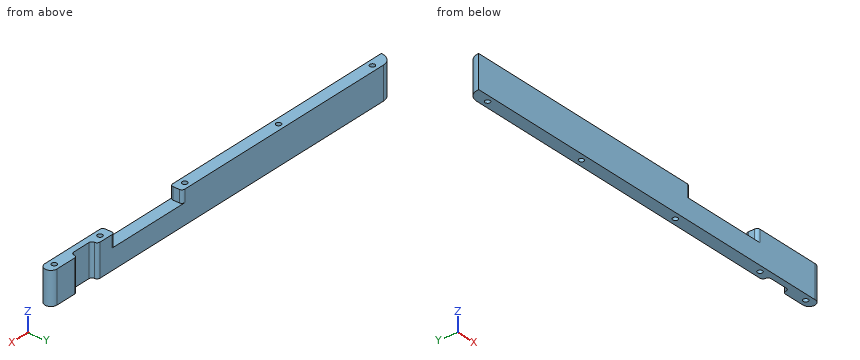
```python
from build123d import *

# Parameters (mm, degrees)
EXTRUDE_854_DEPTH      = 8
SKETCH_2_W             = 20
SKETCH_2_H             = 3
CUT_EXTRUDE_1137_DEPTH = 3
HOLE_WIZARD_1_6_D      = 1.25
SKETCH_7_W             = 6
SKETCH_7_H             = 1.5
CUT_EXTRUDE_2764_DEPTH = 102.181383663
FILLET_2_RADIUS        = 1.5
FILLET_2_LENGTH        = 8
FILLET_3_R             = 0.75


with BuildPart() as part:
    # Model → Extrude 854 (new body)
    with BuildSketch(Plane.XY):
        with BuildLine():
            Line((100.82, 3), (3, 3))
            ThreePointArc((3, 3), (0.878679656, 2.121320344), (0, 0))
            Line((0, 0), (100.82, 0))
            Line((100.82, 0), (100.82, 3))
        make_face()
    extrude(amount=EXTRUDE_854_DEPTH)

    # Эскиз2 → Cut-Extrude 1137 (cut)
    with BuildSketch(Plane.XY.offset(8)):
        with Locations((72.34, 1.5)):
            Rectangle(SKETCH_2_W, SKETCH_2_H)
    extrude(amount=-CUT_EXTRUDE_1137_DEPTH, mode=Mode.SUBTRACT)

    # Резьба М1.6 (through all)
    with Locations(Plane.XY.offset(8)):
        with Locations((4.42, 1.5), (59.84, 1.5), (84.84, 1.5), (98.32, 1.5), (32.13, 1.5)):
            Hole(HOLE_WIZARD_1_6_D / 2)

    # Эскиз7 → Cut-Extrude 2764 (cut, through all)
    with BuildSketch(Plane.XY.offset(8)):
        with Locations((90.37, 2.25)):
            Rectangle(SKETCH_7_W, SKETCH_7_H)
    extrude(amount=-CUT_EXTRUDE_2764_DEPTH, mode=Mode.SUBTRACT)

    # Скругление2: full round fillet: the end face becomes a half cylinder, R = half its width
    fillet_2_face = Plane((100.82, 1.5, 4), x_dir=(0, 0, 1), z_dir=(1, 0, 0))  # on the end face: x along it, z out of the body
    fillet_2_slab = fillet_2_face.offset(-FILLET_2_RADIUS / 2) * Box(FILLET_2_LENGTH, 2 * FILLET_2_RADIUS, FILLET_2_RADIUS, mode=Mode.PRIVATE)  # the body's end, R deep
    fillet_2_round = Plane((99.32, 1.5, 4), x_dir=(1, 0, 0), z_dir=(0, 0, 1)) * Cylinder(FILLET_2_RADIUS, FILLET_2_LENGTH, mode=Mode.PRIVATE)  # its axis R under the face
    add(fillet_2_slab - fillet_2_round, mode=Mode.SUBTRACT)

    # Скругление3
    fillet_3_edges = [part.edges().sort_by_distance(p)[0] for p in [
        (62.34, 0, 6.5),
        (82.34, 0, 6.5),
        (93.37, 1.5, 4),
        (93.37, 3, 4),
        (87.37, 1.5, 4),
        (87.37, 3, 4),
        (82.34, 3, 6.5),
        (62.34, 3, 6.5),
    ]]
    fillet(fillet_3_edges, radius=FILLET_3_R - 0.0001)  # a hair under: the kernel refuses the full size


solid = part.part
```
Geometry check sheet. Reference: the model listing, model coordinates, mm. Round coordinates to 2 decimals unless told otherwise and drop trailing zeros. Order: outer loops, then holes, each group sorted by start corner. A loop starts at its lowest first (then second) coordinate and runs counter-clockwise, first axis right, second up. Notation, with made-up numbers: (39.5, 13) -> (68.5, 13) arc R25 cw to (68.5, 28) -> close; hole circle Ø4 at (11, 19.25). An arc over 180 degrees is marked (long way). Return JSON: item names as keys, results as strings. Group by question number.
Q1. Material ranges on probe 1 along Y at (x, z) = (84.84, 6.25) (3 decimals); probe 2 along X at (y, z) = (1.45, 1); probe 3 along X at (y, z) = (1.15, 2), recorded low to high. Write a range as from..to.
Q2. Section check B-B, the plane x = 90.5. Record the boundary of the cut face in (y, z), plus the area to 3 significant figures.
Q3. Section check A-A, the plane z = 3.75. Count the separate pieces of the cut face and the enclosed holes in it, plus the area to 3 significant figures.
Q4. Gauge pin test, flat ends, axial feed: pin 1 (3.5 mm diameter, centred on x = 90.5, z = 2.5, fed in from +Y); pin 2 (1.2 mm diameter, centred on y = 2, z = 6, fed in from -X); pin 3 (1 mm diameter, centred on x = 84.84, y = 1.5, fed in from -Z). Record the tip position at first contact, or that the pin passes through.
Numbers:
{
 "1": {"probe 1": "0..0.875, 2.125..3", "probe 2": "0.37..3.8, 5.04..31.51, 32.75..59.22, 60.46..84.22, 85.46..97.7, 98.94..100.82", "probe 3": "0.23..3.9, 4.94..31.61, 32.65..59.32, 60.36..84.32, 85.36..97.8, 98.84..100.78"},
 "2": {"outline": "(0, 0) -> (1.5, 0) -> (1.5, 8) -> (0, 8) -> close", "area": "12.0 mm^2"},
 "3": {"separate pieces": "1", "enclosed holes": "5", "area": "284 mm^2"},
 "4": {"pin 1": "y = 1.5", "pin 2": "x = 0.35", "pin 3": "through"}
}
